Build history of the part. All positions in model axes, mm. Face numbers are marked on the shaded views. A direction names the side the tool comes from. Give positions to 0.01 mm unless a question says otherwise; leave off trailing zeros. Write each loop counter-clockwise with the first axis right and the second up, starting at its lowest first coordinate (ties: lowest second). Pieces come first, ordered by that corner, then holes. Notation, with made-up numbers: M -34.5,43 L 6.5,43 A12 ccw 6.5,53 Z; hole C 57.25,62.25 d8. An arc over 180 degrees is marked long. Return JSON: item names as keys, results as strings. Group by question number.
Q1. Pull direction Y, two halves, no side cores. Call the marked faces 5, 6 and 7: +Y half, -Y half, draft (parallel to the pull), parting line (faces both ways), or undercut.
Q2. Tool access for the marked faces 1, 2, 3 and 4: list every direction of +Z, -Z, +X, -X, +Y, -Y with a clear straight run to the whole face (end or side of a thin tool).
Q3. Flat gauge pins, fed straight in: pin 1 Ø2.5 at (y, z) = (0.5, 2.5) entering from -X (3 decimals); pin 2 Ø2.5 at (x, z) = (1, 4) entering from -Y (3 decimals); pin 3 Ø1 at (x, y) = (-8, 1.5) entering from -Z; pin 4 Ø1 at (y, z) = (1.5, 5.5) entering from +X (3 decimals). Where does each tip first touch, or does it go through?
Q4. Band-saw the part on A-A, the plane x = 0. Give the cut face in (y, z) (3 decimals), then the cut area to 3 significant figures.
Q5. Wall check: probe 1 along Y at (x, z) = (0, 4) (3 decimals); probe 2 along Y at (x, z) = (11, 5); probe 3 along X at (y, z) = (-6.5, 2) (1 decimal). Give the ranges that are in metal, low to high.
Q6. Band-saw the part on B-B, the plane y = 0. Give the cut face in (x, z) (3 decimals), then the cut area to 3 significant figures.
from build123d import *

# Parameters (mm, degrees)
SKETCH1_R           = 4.15
BOSS_EXTRUDE1_DEPTH = 6.35


with BuildPart() as part:
    # Sketch1 → Boss-Extrude1 (new body)
    with BuildSketch(Plane.XY):
        Polygon((-14.425, 9.56), (-14.425, 2.56), (-8.075, 2.56), (-8.075, -2.505147932), (-14.425, -2.505147932), (-14.425, -9.56), (-2.5325, -9.56), (-2.5325, -6.385), (0, -6.385), (2.5325, -6.385), (2.5325, -9.56), (14.425, -9.56), (14.425, -2.505147932), (8.075, -2.505147932), (8.075, 2.56), (14.425, 2.56), (14.425, 9.56), align=None)
        Circle(SKETCH1_R, mode=Mode.SUBTRACT)
    extrude(amount=BOSS_EXTRUDE1_DEPTH)


solid = part.part
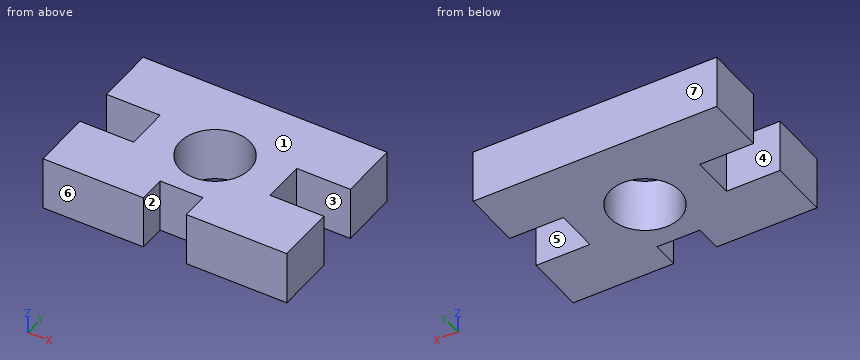
From the geometry:
{
 "1": {"face 5": "undercut", "face 6": "-Y half", "face 7": "+Y half"},
 "2": {"face 1": "+Z, +X, -X, +Y, -Y", "face 2": "+Z, -Z, -Y", "face 3": "+Z, -Z, +X", "face 4": "+Z, -Z, -X"},
 "3": {"pin 1": "stops at x = -8.075", "pin 2": "stops at y = -6.385", "pin 3": "stops at z = 0", "pin 4": "stops at x = 8.075"},
 "4": {"outline": "M -6.385,0 L -4.15,0 L -4.15,6.35 L -6.385,6.35 Z; M 4.15,0 L 9.56,0 L 9.56,6.35 L 4.15,6.35 Z", "area": "48.5 mm^2"},
 "5": {"probe 1": "y = -6.385 to -4.15, 4.15 to 9.56", "probe 2": "y = -9.56 to -2.51, 2.56 to 9.56", "probe 3": "x = -14.4 to -2.5, 2.5 to 14.4"},
 "6": {"outline": "M -8.075,0 L -4.15,0 L -4.15,6.35 L -8.075,6.35 Z; M 4.15,0 L 8.075,0 L 8.075,6.35 L 4.15,6.35 Z", "area": "49.8 mm^2"}
}
